Design review of the part shown in the three views and the two pictorial views. Dimensions are in mm from the part's minimum x, y and z. Coordinates: 2 decimals unless noted, no trailing zeros. Loops run counter-clockwise (first coordinate to the right, second up) from the corner with the lowest first, then second, coordinate; pieces in that order, holes last. Notation, with made-up numbers: (25.5, 7) - (35.5, 7) arc R11 ccw to (35.5, 19) - close; hole circle Ø11 at (40, 30.5). An arc over 180 degrees is marked (long way). One line per question, with ' | ' between items.
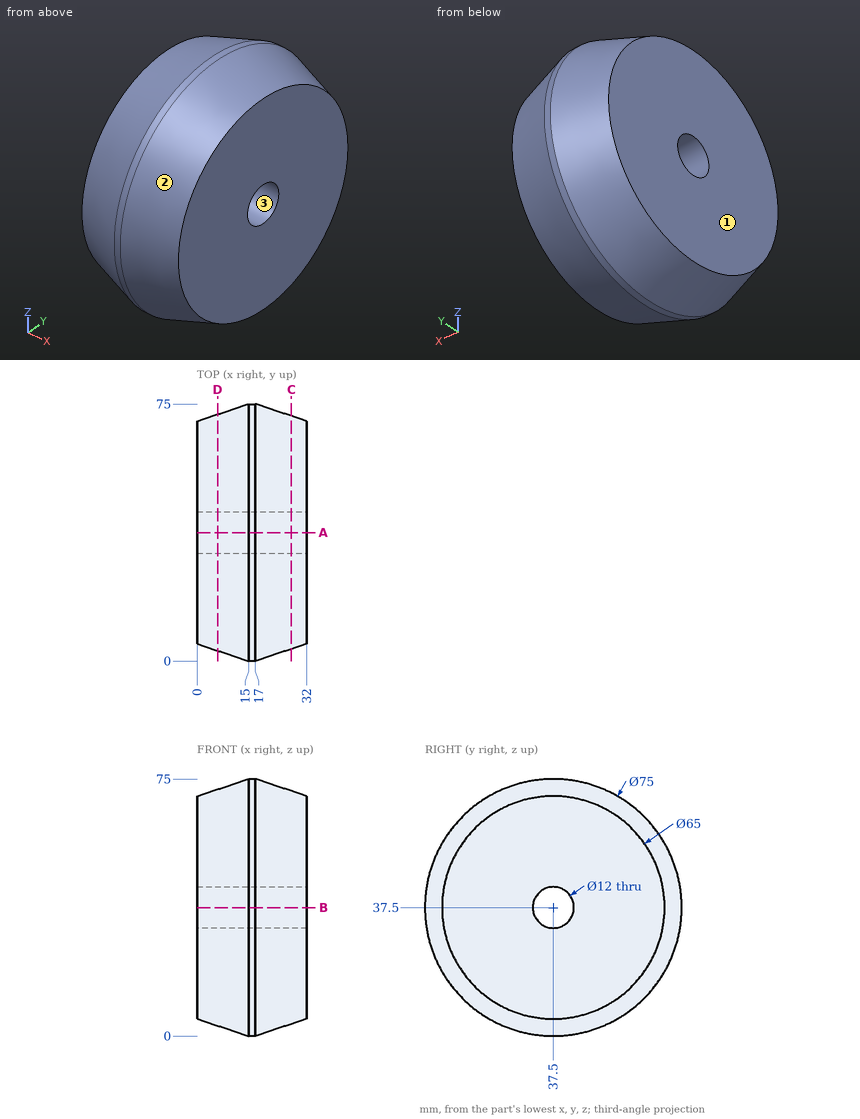
Q1. Take a section at A-A (y = 37.5). Give the boundary of the cut face in (x, z), plus the area to 3 significant figures.
Returned:
outline: (0, 5) - (15, 0) - (17, 0) - (32, 5) - (32, 31.5) - (0, 31.5) - close; (0, 43.5) - (32, 43.5) - (32, 70) - (17, 75) - (15, 75) - (0, 70) - close | area: 1,870 mm²
Q2. Draft analysis for pull direction Y (two halves, no side actions). For the marked faces 1, 2 and 3, state which applies: +Y half, -Y half, draft (parallel to the pull), parting line (faces both ways), or undercut.
Returned:
face 1: draft | face 2: parting line | face 3: undercut
Q3. Take a section at C-C (x = 27.5). Give the boundary of the cut face in (y, z).
Returned:
outline: circle Ø68 at (37.5, 37.5); hole circle Ø12 at (37.5, 37.5)
Q4. To check wall thickness, follow line 1 along Y through (x, z) = (8, 37.5); line 2 along Y through (x, z) = (3, 36.5); line 3 along Z through (x, y) = (9.5, 33). State the ranges of each line that lie inside material, in increasing order.
Returned:
line 1: y = 2.33 to 31.5, 43.5 to 72.67 | line 2: y = 4.01 to 31.58, 43.42 to 70.99 | line 3: z = 2.12 to 33.53, 41.47 to 72.88
Q5. Take a section at D-D (x = 6). Give the boundary of the cut face in (y, z).
Returned:
outline: circle Ø69 at (37.5, 37.5); hole circle Ø12 at (37.5, 37.5)
Q6. For pin 1 (11 mm diameter, centred on y = 37.5, z = 37.5, fed in from +X); pin 2 (4 mm diameter, centred on x = 22.5, z = 64, fed in from -Y); pin 3 (1 mm diameter, centred on x = 17, y = 48.5, fed in from -Z); pin 4 (6 mm diameter, centred on x = 17.5, z = 13, fed in from +Y), all flat-tipped, find the tip position at first contact; note any pin that passes through.
Returned:
pin 1: passes through | pin 2: stops at y = 11.37 | pin 3: stops at z = 1.5 | pin 4: stops at y = 68.2
